Autodesk Inventor part; units mm, degrees
ref_plane "YZ Plane" through (0, 0, 0) normal (1, 0, 0) x (0, 1, 0)
ref_plane "XZ Plane" through (0, 0, 0) normal (0, 1, 0) x (-1, 0, 0)
ref_plane "XY Plane" through (0, 0, 0) normal (0, 0, 1) x (1, 0, 0)
sketch "Sketch1" plane through (0, 0, 0) normal (1, 0, 0) x (0, 1, 0)
  line L0 (-216, 200) -> (216, 200)
  line L1 (216, 200) -> (216, -200)
  line L2 (216, -200) -> (-216, -200)
  line L3 (-216, -200) -> (-216, 200)
  line L4 (-216, 200) -> (216, -200) construction
  line L5 (216, 200) -> (-216, -200) construction
  point P0 (0, 0)
  dimension "d0" = 432
  dimension "d1" = 400
extrude "Extrusion1" add sketch "Sketch1" along normal mid plane 3
sketch "Sketch2" plane through (1.5, 0, 0) normal (1, 0, 0) x (0, 0, -1)
  line L0 (200, -216) -> (200, 216)
  line L1 (200, -158) -> (138, -158)
  line L2 (138, -158) -> (138, -128)
  line L3 (138, -128) -> (-72, -128)
  line L4 (-72, -128) -> (-72, 128)
  line L5 (-72, 128) -> (138, 128)
  line L6 (138, 128) -> (138, 158)
  line L7 (138, 158) -> (200, 158)
  line L8 (-200, -216) -> (200, -216)
  line L9 (200, 216) -> (-200, 216)
  point P0 (0, 0)
  dimension "d4" = 58
  dimension "d5" = 58
  dimension "d6" = 62
  dimension "d7" = 30
  dimension "d8" = 210
extrude "Extrusion2" cut sketch "Sketch2" against normal blind 3
sketch "Sketch3" plane through (1.5, 0, 0) normal (1, 0, 0) x (0, 0, -1)
  circle A0 centre (3, 199) radius 3
  circle A1 centre (103, 199) radius 3
  circle A2 centre (-97, 199) radius 3
  circle A3 centre (-97, -199) radius 3
  circle A4 centre (3, -199) radius 3
  circle A5 centre (103, -199) radius 3
  line L0 (-200, 216) -> (-200, -216)
  line L1 (200, 216) -> (-200, 216)
  line L2 (-200, -216) -> (200, -216)
  point P0 (0, 0)
  dimension "d13" = 103
  dimension "d14" = 17
  dimension "d15" = 6
  dimension "d16" = 100
  dimension "d17" = 100
  dimension "d18" = 17
  dimension "d19" = 100
extrude "Extrusion3" cut sketch "Sketch3" against normal blind 3
sketch "Sketch4" plane through (1.5, 0, 0) normal (1, 0, 0) x (0, 0, -1)
  circle A0 centre (-183, -113) radius 2.5
  circle A1 centre (-183, -13) radius 2.5
  arc A2 (-183, 79.5) -> (-183, 94.5) centre (-183, 87) ccw
  line L0 (-183, 94.5) -> (-194, 94.5)
  line L1 (-194, 79.5) -> (-194, 94.5)
  line L2 (-183, 79.5) -> (-194, 79.5)
  circle A3 centre (-183, 87) radius 2.5
  point P0 (0, 0)
hole "Hole1" at (1.5, -113, 183) at (1.5, -13, 183) at (1.5, 87, 183) direction (-1, 0, 0) diameter 6 depth 14.2 tip angle 118
equation "\"d5\" = d4"
properties part number "HCMUTE-CDT23-KXL_A04" material "PMMA Plastic"
Input: part model. Units: mm. Frame: model coordinates. Coordinates: 2 decimals unless noted, no trailing zeros. Loops run counter-clockwise (first coordinate to the right, second up) from the corner with the lowest first, then second, coordinate; pieces in that order, holes last. Notation, with made-up numbers: (-35.5, -22) -> (-19.5, -22) arc R7 cw to (-19.5, -16) -> close; hole circle Ø6 at (9, 84.25). An arc over 180 degrees is marked (long way). Write each question's results on one line, items separated by ' | '. Start each with the question number.
Q1. Section D-D, the plane y = -44. Return the cut outline in (x, z).
Q2. Section B-B, the plane x = -0.3. State how many separate pieces and enclosed holes the cut face has, plus the area to 3 significant figures.
Q3. Section C-C, the plane z = -41. Return the cut outline in (x, y).
Q4. Ray query, line 1 (Z direction, x = -0.2, y = -199); line 2 (Y direction, x = 0.75, z = -103); line 3 (Y direction, x = -0.1, z = 183). Return the intervals inside material, ascending. Write a range as from..to.
Q5. Pin query (flat end, axial travel): pin 1 (0.9 mm diameter, centred on x = -0.5, y = 143, fed in from -Z); pin 2 (1 mm diameter, centred on x = 1, y = -99, fed in from -Z). Return the tip coordinate at first contact, or that it passes through.
Q6. Section A-A, the plane z = -149. Return the cut outline in (x, y), plus the area to 3 significant figures.
Found:
1) outline: (-1.5, 72) -> (1.5, 72) -> (1.5, 200) -> (-1.5, 200) -> close
2) separate pieces: 1 | enclosed holes: 9 | area: 99,200 mm2
3) outline: (-1.5, -216) -> (1.5, -216) -> (1.5, -128) -> (-1.5, -128) -> close; (-1.5, 128) -> (1.5, 128) -> (1.5, 216) -> (-1.5, 216) -> close
4) line 1: -200..-106, -100..-6, 0..94, 100..200 | line 2: -216..-202, -196..-128, 128..196, 202..216 | line 3: -216..-116, -110..-16, -10..84, 90..216
5) pin 1: z = -138 | pin 2: z = 72
6) outline: (-1.5, -216) -> (1.5, -216) -> (1.5, -158) -> (-1.5, -158) -> close; (-1.5, 158) -> (1.5, 158) -> (1.5, 216) -> (-1.5, 216) -> close | area: 348 mm2
